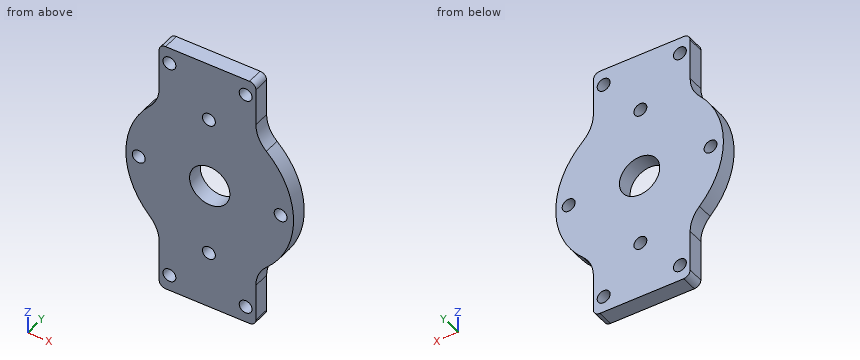
```python
from build123d import *

# Parameters (mm, degrees)
Y_KSEKLIK_EKSTR_ZYON1_DEPTH = 2.5
IZIM2_R                     = 2
KES_EKSTR_ZYON1_DEPTH       = 27
DAIRESEL_KAPLAMA1_COUNT     = 2
DAIRESEL_KAPLAMA1_ANGLE     = 90
IZIM3_R                     = 6.25
KES_EKSTR_ZYON2_DEPTH       = 27
IZIM4_R                     = 2
KES_EKSTR_ZYON3_DEPTH       = 27
RADYUS1_R                   = 2


with BuildPart() as part:
    # Çizim1 → Yükseklik-Ekstrüzyon1 (new, symmetric)
    with BuildSketch(Plane(origin=(0, 0, 0), x_dir=(1, 0, 0), z_dir=(0, 1, 0))):
        with BuildLine():
            Line((-15.675675676, 40), (-15.675675676, 25.234097539))
            ThreePointArc((-15.675675676, 25.234097539), (-16.420371215, 21.447365526), (-18.543543544, 18.224626))
            ThreePointArc((-18.543543544, 18.224626), (-26, 0), (-18.543543544, -18.224626))
            ThreePointArc((-18.543543544, -18.224626), (-16.420371215, -21.447365526), (-15.675675676, -25.234097539))
            Line((-15.675675676, -25.234097539), (-15.675675676, -40))
            Line((-15.675675676, -40), (14.324324324, -40))
            Line((14.324324324, -40), (14.324324324, -26.539164383))
            ThreePointArc((14.324324324, -26.539164383), (15.170976096, -22.512228052), (17.567567568, -19.167174277))
            ThreePointArc((17.567567568, -19.167174277), (26, 0), (17.567567568, 19.167174277))
            ThreePointArc((17.567567568, 19.167174277), (15.170976096, 22.512228052), (14.324324324, 26.539164383))
            Line((14.324324324, 26.539164383), (14.324324324, 40))
            Line((14.324324324, 40), (-15.675675676, 40))
        make_face()
    extrude(amount=Y_KSEKLIK_EKSTR_ZYON1_DEPTH, both=True)

    # Çizim2 → Kes-Ekstrüzyon1 (cut)
    with BuildSketch(Plane(origin=(0, 2.5, 0), x_dir=(1, 0, 0), z_dir=(0, 1, 0))):
        with Locations(Location((-22, 0, 0), (0, 0, 270))):
            Circle(IZIM2_R)
        with Locations(Location((22, 0, 0), (0, 0, 270))):
            Circle(IZIM2_R)
    kes_ekstr_zyon1 = extrude(amount=-KES_EKSTR_ZYON1_DEPTH, mode=Mode.SUBTRACT)

    # Dairesel Kaplama1: Kes-Ekstrüzyon1 ×2 about axis
    dairesel_kaplama1_axis = Axis((-0.246697988, 0, 0), (0, 1, 0))
    for i in range(1, DAIRESEL_KAPLAMA1_COUNT):
        add(kes_ekstr_zyon1.rotate(dairesel_kaplama1_axis, i * DAIRESEL_KAPLAMA1_ANGLE / (DAIRESEL_KAPLAMA1_COUNT - 1)), mode=Mode.SUBTRACT)

    # Çizim3 → Kes-Ekstrüzyon2 (cut)
    with BuildSketch(Plane(origin=(0, 2.5, 0), x_dir=(1, 0, 0), z_dir=(0, 1, 0))):
        with Locations(Location((0, 0, 0), (0, 0, 270))):
            Circle(IZIM3_R)
    extrude(amount=-KES_EKSTR_ZYON2_DEPTH, mode=Mode.SUBTRACT)

    # Çizim4 → Kes-Ekstrüzyon3 (cut)
    with BuildSketch(Plane(origin=(0, 2.5, 0), x_dir=(1, 0, 0), z_dir=(0, 1, 0))):
        with Locations(Location((-12.5, 35, 0), (0, 0, 270))):
            Circle(IZIM4_R)
        with Locations(Location((11.148648649, 35, 0), (0, 0, 270))):
            Circle(IZIM4_R)
    kes_ekstr_zyon3 = extrude(amount=-KES_EKSTR_ZYON3_DEPTH, mode=Mode.SUBTRACT)

    # Aynalama1: Kes-Ekstrüzyon3 across plane
    add(kes_ekstr_zyon3.mirror(Plane.XY), mode=Mode.SUBTRACT)

    # Radyus1
    radyus1_edges = [part.edges().sort_by_distance(p)[0] for p in [
        (-15.675675676, 0, -40),
        (14.324324324, 0, -40),
        (14.324324324, 0, 40),
        (-15.675675676, 0, 40),
    ]]
    fillet(radyus1_edges, radius=RADYUS1_R)


solid = part.part
```
Read the model definition and answer for the solid it produces. Units are mm, in the model's axes. Coordinates: 2 decimals unless noted, no trailing zeros. Order: outer loops, then holes, each group sorted by start corner. A loop starts at its lowest first (then second) coordinate and runs counter-clockwise, first axis right, second up. Notation, with made-up numbers: (24.25, -18.75) - (39.25, -18.75) arc R17 cw to (39.25, 3.25) - close; hole circle Ø7 at (39, 13). An arc over 180 degrees is marked (long way). Answer as a JSON object with one key per item and string values. Group by question number.
Item 1: Section C-C (x = 0) is taken. Give the vertices of the cut face in (y, z).
Item 2: Consider probe 1 along X at (y, z) = (0.55, -35); probe 2 along Z at (x, y) = (-11, -1.6); probe 3 along Z at (x, y) = (10.5, 0.05). Determine where each line is inside the solid, lowest interval first. Write a range as from..to.
Item 3: Section B-B (x = -12.5) is taken. Give the vertices of the cut face in (y, z), plus the area to 3 significant figures.
Item 4: Section A-A (z = -35) is taken. Give the vertices of the cut face in (x, y).
Item 5: Flat-ended cylindrical pins translate along their axes: P1, Ø1, axis at y = -1.5, z = -8.5, coming from the +X side; P2, Ø2.5, axis at x = -12.5, z = 35, coming from the +Y side; P3, Ø5, axis at x = 22, z = 0, coming from the -Y side; P4, Ø1.5, axis at y = 0, z = -31, coming from the -X side. Find the tip coordinate at first contact, or state that the pin passes through.
Item 6: Section D-D (y = 1.35) is taken. State how many separate pieces and enclosed holes the cut face has, plus the area to 3 significant figures.
Results are:
{
 "1": {"outline": "(-2.5, -40) - (2.5, -40) - (2.5, -24.23) - (-2.5, -24.23) - close; (-2.5, -20.26) - (2.5, -20.26) - (2.5, -6.25) - (-2.5, -6.25) - close; (-2.5, 6.25) - (2.5, 6.25) - (2.5, 19.77) - (-2.5, 19.77) - close; (-2.5, 23.74) - (2.5, 23.74) - (2.5, 40) - (-2.5, 40) - close"},
 "2": {"probe 1": "x = -15.68..-14.5, -10.5..9.15, 13.15..14.32", "probe 2": "z = -40..-36.32, -33.68..33.68, 36.32..40", "probe 3": "z = -40..-36.89, -33.11..33.11, 36.89..40"},
 "3": {"outline": "(-2.5, -40) - (2.5, -40) - (2.5, -37) - (-2.5, -37) - close; (-2.5, -33) - (2.5, -33) - (2.5, 33) - (-2.5, 33) - close; (-2.5, 37) - (2.5, 37) - (2.5, 40) - (-2.5, 40) - close", "area": "360 mm^2"},
 "4": {"outline": "(-15.68, -2.5) - (-14.5, -2.5) - (-14.5, 2.5) - (-15.68, 2.5) - close; (-10.5, -2.5) - (9.15, -2.5) - (9.15, 2.5) - (-10.5, 2.5) - close; (13.15, -2.5) - (14.32, -2.5) - (14.32, 2.5) - (13.15, 2.5) - close"},
 "5": {"P1": "stops at x = 24.74", "P2": "passes through", "P3": "stops at y = -2.5", "P4": "stops at x = -15.68"},
 "6": {"separate pieces": "1", "enclosed holes": "9", "area": "2,840 mm^2"}
}
